Design review of the part built by this model. Coordinates are the model's own, in mm. A direction names the side the tool comes from. Give positions to 0.01 mm unless a question says otherwise; leave off trailing zeros. Order: outer loops, then holes, each group sorted by start corner. A loop starts at its lowest first (then second) coordinate and runs counter-clockwise, first axis right, second up. Notation, with made-up numbers: (31.25, 3) -> (81.25, 3) arc R38 ccw to (81.25, 41) -> close; hole circle Ø5 at (-35, 88). An arc over 180 degrees is marked (long way). Use a Markdown table: item, result. Add a question column.
```python
from build123d import *

# Parameters (mm, degrees)
F1_DEPTH = 28.575
F2_W     = 16.383
F2_H     = 6.985
F3_DEPTH = 3.175
F4_R     = 1.5875


with BuildPart() as f1:
    # F0 (on Top) → F1 (new body)
    with BuildSketch(Plane.XY):
        with BuildLine():
            Line((-15.24, 40.005), (-15.24, 28.956))
            Line((-15.24, 28.956), (-27.305, 28.956))
            ThreePointArc((-27.305, 28.956), (-38.53032, 24.30632), (-43.18, 13.081))
            Line((-43.18, 13.081), (-43.18, -13.081))
            ThreePointArc((-43.18, -13.081), (-38.53032, -24.30632), (-27.305, -28.956))
            Line((-27.305, -28.956), (27.305, -28.956))
            ThreePointArc((27.305, -28.956), (38.53032, -24.30632), (43.18, -13.081))
            Line((43.18, -13.081), (43.18, 13.081))
            ThreePointArc((43.18, 13.081), (38.53032, 24.30632), (27.305, 28.956))
            Line((27.305, 28.956), (15.24, 28.956))
            Line((15.24, 28.956), (15.24, 40.005))
            Line((15.24, 40.005), (-15.24, 40.005))
        make_face()
        with BuildLine():
            Line((12.065, 25.781), (27.305, 25.781))
            ThreePointArc((27.305, 25.781), (36.285256, 22.061256), (40.005, 13.081))
            Line((40.005, 13.081), (40.005, -13.081))
            ThreePointArc((40.005, -13.081), (36.285256, -22.061256), (27.305, -25.781))
            Line((27.305, -25.781), (-27.305, -25.781))
            ThreePointArc((-27.305, -25.781), (-36.285256, -22.061256), (-40.005, -13.081))
            Line((-40.005, -13.081), (-40.005, 13.081))
            ThreePointArc((-40.005, 13.081), (-36.285256, 22.061256), (-27.305, 25.781))
            Line((-27.305, 25.781), (-12.065, 25.781))
            Line((-12.065, 25.781), (-12.065, 36.83))
            Line((-12.065, 36.83), (12.065, 36.83))
            Line((12.065, 36.83), (12.065, 25.781))
        make_face(mode=Mode.SUBTRACT)
    extrude(amount=F1_DEPTH)

    # F2 (on face) → F3 (cut, through all)
    with BuildSketch(Plane(origin=(0, 40.005, 0), x_dir=(-1, 0, 0), z_dir=(0, 1, 0))):
        with Locations((0, 17.8435)):
            Rectangle(F2_W, F2_H)
    extrude(amount=-F3_DEPTH, mode=Mode.SUBTRACT)

    # F4
    f4_edges = [f1.edges().sort_by_distance(p)[0] for p in [
        (-12.065, 25.781, 14.2875),
        (-12.065, 36.83, 14.2875),
        (12.065, 25.781, 14.2875),
        (12.065, 36.83, 14.2875),
        (15.24, 40.005, 14.2875),
        (-15.24, 40.005, 14.2875),
    ]]
    fillet(f4_edges, radius=F4_R)


with BuildPart() as f5_1:
    # F5: copy of F1
    add(f1.part)


solid = f1.part
```
1) Add section A-A (x = 22.5). Give the boundary of the cut face in (y, z) (3 decimals), then the cut area to 3 significant figures.
2) For L1, parallel to Y at x = 9.5, z = 14.25 (3 decimals); L2, parallel to X at y = -9, z = 26.75 (3 decimals); L3, parallel to X at y = 37.5, z = 19.25, list the stretches that pass through material, from the lowest coordinate up. Write a range as [from, to].
3) The part is to be moulded in two halves that separate along Y. For faces 1 (the flat face through (-13, 26.1, 0)), 2 (the cylindrical face through (-36.383, 21.962, 14.087)), 3 (the cylindrical face through (38.406, -24.429, 14.087)), say which applies: +Y half, -Y half, draft (parallel to the pull), parting line (faces both ways), or undercut.
4) Machinability: for faces 4 (the flat face through (0, 38, 21.336)), 5 (the cylindrical face through (36.186, 22.159, 14.087)), 6 (the flat face through (15.24, 34, 14)), which of the approach directions +Z, -Z, +X, -X, +Y, -Y give a long, thin tool a straight path to every point of the face, cutting with its end or side? Answer none if there is none.
5) Insertion check: pin 1 (2.5 mm diameter, centred on y = 32, z = 19.5, fed in from -X); pin 2 (6 mm diameter, centred on y = 29.5, z = 21, fed in from -X); pin 3 (6 mm diameter, centred on x = 19, z = 9, fed in from +Y); pin 4 (12 mm diameter, centred on x = -29, y = -12.5, fed in from +Z). Each pin has a flat end and moves straight along its axis. Give the tip position at first contact, or say it passes through.
6) Add section B-B (y = -4.5). Give the boundary of the cut face in (x, z) (3 decimals).
7) Add section D-D (x = 2). Give the boundary of the cut face in (y, z) (3 decimals), then the cut area to 3 significant figures.
Worked answers:
| question | item | result |
|---|---|---|
| 1 | outline | (-28.956, 0) -> (-25.781, 0) -> (-25.781, 28.575) -> (-28.956, 28.575) -> close; (25.781, 0) -> (28.956, 0) -> (28.956, 28.575) -> (25.781, 28.575) -> close |
| 1 | area | 181 mm^2 |
| 2 | L1 | [-28.956, -25.781], [36.83, 40.005] |
| 2 | L2 | [-43.18, -40.005], [40.005, 43.18] |
| 2 | L3 | [-15.24, -8.19], [8.19, 15.24] |
| 3 | face 1 | draft |
| 3 | face 2 | undercut |
| 3 | face 3 | -Y half |
| 4 | face 4 | +Y |
| 4 | face 5 | +Z, -Z |
| 4 | face 6 | +Z, -Z, +X, +Y |
| 5 | pin 1 | x = -15.24 |
| 5 | pin 2 | x = -35.79 |
| 5 | pin 3 | y = 28.96 |
| 5 | pin 4 | through |
| 6 | outline | (-43.18, 0) -> (-40.005, 0) -> (-40.005, 28.575) -> (-43.18, 28.575) -> close; (40.005, 0) -> (43.18, 0) -> (43.18, 28.575) -> (40.005, 28.575) -> close |
| 7 | outline | (-28.956, 0) -> (-25.781, 0) -> (-25.781, 28.575) -> (-28.956, 28.575) -> close; (36.83, 0) -> (40.005, 0) -> (40.005, 14.351) -> (36.83, 14.351) -> close; (36.83, 21.336) -> (40.005, 21.336) -> (40.005, 28.575) -> (36.83, 28.575) -> close |
| 7 | area | 159 mm^2 |
